from build123d import *

# Parameters (mm, degrees)
SKETCH1_W                = 76.2
SKETCH1_H                = 45.72
BOSS_EXTRUDE1_DEPTH      = 0.8255
SKETCH2_R                = 10.16
BOSS_EXTRUDE2_DEPTH      = 5.08
SKETCH3_W                = 6.731
SKETCH3_H                = 6.858
BOSS_EXTRUDE3_DEPTH      = 1.651
SKETCH4_R                = 2.54
BOSS_EXTRUDE4_DEPTH      = 7.62
BOSS_EXTRUDE5_DEPTH      = 5.969
BOSS_EXTRUDE5_DEPTH_BACK = 2.54
SKETCH5_W                = 4.826
SKETCH5_H                = 6.096
SKETCH6_W                = 7.366
SKETCH6_H                = 8.89
BOSS_EXTRUDE6_DEPTH      = 3.429
M2_CLEARANCE_HOLE1_D     = 2.4
FILLET1_R                = 2.54


with BuildPart() as part:
    # Sketch1 → Boss-Extrude1 (new, symmetric)
    with BuildSketch(Plane(origin=(0, 0, 0), x_dir=(1, 0, 0), z_dir=(0, 1, 0))):
        Rectangle(SKETCH1_W, SKETCH1_H)
    extrude(amount=BOSS_EXTRUDE1_DEPTH, both=True)

    # Sketch2 → Boss-Extrude2 (add)
    with BuildSketch(Plane.XZ.offset(0.8255)):
        with Locations(Location((-19.05, 10.16, 0), (0, 0, 90))):
            Circle(SKETCH2_R)
    extrude(amount=BOSS_EXTRUDE2_DEPTH)

    # Sketch3 → Boss-Extrude3 (add)
    with BuildSketch(Plane.ZY.offset(38.1)):
        with Locations((12.7, 0.8255)):
            Rectangle(SKETCH3_W, SKETCH3_H)
    extrude(amount=BOSS_EXTRUDE3_DEPTH)

    # Sketch4 → Boss-Extrude4 (add)
    with BuildSketch(Plane.ZY.offset(39.751)):
        with Locations(Location((12.7, 0.8255, 0), (0, 0, 180))):
            Circle(SKETCH4_R)
    extrude(amount=BOSS_EXTRUDE4_DEPTH)

    # Sketch5 → Boss-Extrude5 (add, two sides: drawn at the far end of the back side and taken through both)
    with BuildSketch(Plane(origin=(0, 0.8255, 0), x_dir=(1, 0, 0), z_dir=(0, 1, 0)).offset(-BOSS_EXTRUDE5_DEPTH_BACK)):
        with Locations((31.75, -13.335)):
            Rectangle(SKETCH5_W, SKETCH5_H)
        with Locations((31.75, -5.969)):
            Rectangle(SKETCH5_W, SKETCH5_H)
    extrude(amount=BOSS_EXTRUDE5_DEPTH + BOSS_EXTRUDE5_DEPTH_BACK)

    # Sketch6 → Boss-Extrude6 (add)
    with BuildSketch(Plane(origin=(0, 0.8255, 0), x_dir=(1, 0, 0), z_dir=(0, 1, 0))):
        with Locations((34.417, 10.16)):
            Rectangle(SKETCH6_W, SKETCH6_H)
    extrude(amount=BOSS_EXTRUDE6_DEPTH)

    # M2 Clearance Hole1 (through all)
    with Locations(Plane(origin=(0, 0.8255, 0), x_dir=(1, 0, 0), z_dir=(0, 1, 0))):
        with Locations((-34.29, 19.05), (34.29, 19.05), (-34.29, -19.05), (34.29, -19.05)):
            Hole(M2_CLEARANCE_HOLE1_D / 2)

    # Fillet1
    fillet1_edges = [part.edges().sort_by_distance(p)[0] for p in [
        (38.1, 0, 22.86),
        (-38.1, 0, 22.86),
        (-38.1, 0, -22.86),
        (38.1, 0, -22.86),
    ]]
    fillet(fillet1_edges, radius=FILLET1_R)


solid = part.part
Build history of the part. All positions in model axes, mm. A direction names the side the tool comes from. Coordinates: 2 decimals unless noted, no trailing zeros. Order: outer loops, then holes, each group sorted by start corner. A loop starts at its lowest first (then second) coordinate and runs counter-clockwise, first axis right, second up. Notation, with made-up numbers: M -27.75,74.25 L -18.75,74.25 A29 ccw -18.75,96.25 Z; hole C 46.5,-30.5 d7. An arc over 180 degrees is marked long. One line per question, with ' | ' between items. Start each with the question number.
Q1. 3-axis set-ups, long thin cutter, end or side, ignore diameter. For faces 1 (the face through (-39, 1, 9.334)), 2 (the face through (-38.1, 3, 13)), 3 (the face through (34.163, 4, 6)), 4 (the face through (-22.1, -3.33, 19.85)): which of +Z, -Z, +X, -X, +Y, -Y reach the whole face in a straight line?
Q2. Saw through at D-D (y = -3.75). List the corners of the cut face in (x, z).
Q3. Saw through at C-C (z = -7). List the corners of the cut face in (x, y).
Q4. Two-plate mould, pull along X, no slides. Class faces 5 (the face through (-38.1, -2, 13)), 6 (the face through (29.337, 4, 6)), 7 (the face through (32, 6.794, 6)): +X half, -X half, draft (parallel to the pull), parting line (faces both ways), or undercut.
Q5. Probe L1, parallel to Z at x = -34.29, y = -0.05; L2, parallel to X at y = 0.3, z = -19.05; L3, parallel to Y at x = 6.5, z = -19.5. List the from-to ranges inside material, lowest first. Write a range as from..to.
Q6. Saw through at B-B (x = -19.05). List the corners of the cut face in (y, z).
Q7. Flat gauge pins, fed straight in: pin 1 Ø0.5 at (y, z) = (0, -7.5) entering from -X; pin 2 Ø0.5 at (x, y) = (-39, 0.5) entering from +Z; pin 3 Ø1 at (y, z) = (3, -10) entering from -X; pin 4 Ø5 at (x, y) = (25, 4.5) entering from -Z. Where does each tip first touch, or does it go through?
Q8. Saw through at A-A (z = 19.05). List the corners of the cut face in (x, y), then the cut area to 3 significant figures.
Check values:
1) face 1: -Z, -X, +Y, -Y | face 2: +Z, -Z, +Y | face 3: +Z, +X, +Y | face 4: -Y
2) outline: C -19.05,10.16 d20.32
3) outline: M -38.1,-0.83 L 38.1,-0.83 L 38.1,4.25 L 30.73,4.25 L 30.73,0.83 L -38.1,0.83 Z
4) face 5: undercut | face 6: -X half | face 7: draft
5) L1: z = -22.86..-20.25, -17.85..17.85, 20.25..22.86 | L2: x = -38.1..-35.49, -33.09..33.09, 35.49..38.1 | L3: y = -0.83..0.83
6) outline: M -5.91,0 L -0.83,0 L -0.83,-22.86 L 0.83,-22.86 L 0.83,22.86 L -0.83,22.86 L -0.83,20.32 L -5.91,20.32 Z
7) pin 1: stops at x = -38.1 | pin 2: stops at z = 16.07 | pin 3: stops at x = 30.73 | pin 4: passes through
8) outline: M -38.1,-0.83 L -35.49,-0.83 L -35.49,0.83 L -38.1,0.83 Z; M -33.09,-0.83 L -23.97,-0.83 L -23.97,-5.91 L -14.13,-5.91 L -14.13,-0.83 L 33.09,-0.83 L 33.09,0.83 L -33.09,0.83 Z; M 35.49,-0.83 L 38.1,-0.83 L 38.1,0.83 L 35.49,0.83 Z | area: 168 mm2
